from build123d import *

# Parameters (mm, degrees)
F0_R     = 50
F1_DEPTH = 6
F2_R     = 3
F3_DEPTH = 6.001
F4_R     = 4
F5_DEPTH = 6.001


with BuildPart() as f1:
    # F0 (on Front) → F1 (new body)
    with BuildSketch(Plane.XZ):
        Circle(F0_R)
    extrude(amount=F1_DEPTH)

    # F2 (on face) → F3 (cut, through all)
    with BuildSketch(Plane.XZ.offset(6)):
        Circle(F2_R)
    extrude(amount=-F3_DEPTH, mode=Mode.SUBTRACT)

    # F4 (on face) → F5 (cut, through all)
    with BuildSketch(Plane.XZ.offset(6)):
        with Locations((0, 38)):
            Circle(F4_R)
        with Locations((-22.33584, -30.742646)):
            Circle(F4_R)
        with Locations((-36.140148, 11.742646)):
            Circle(F4_R)
        with Locations((22.33584, -30.742646)):
            Circle(F4_R)
        with Locations((36.140148, 11.742646)):
            Circle(F4_R)
    extrude(amount=-F5_DEPTH, mode=Mode.SUBTRACT)


solid = f1.part
Verification items for the finished model (mm, model axes). Coordinates: 2 decimals unless noted, no trailing zeros. Order: outer loops, then holes, each group sorted by start corner. A loop starts at its lowest first (then second) coordinate and runs counter-clockwise, first axis right, second up. Notation, with made-up numbers: (-35.5, 3.25) -> (-17.5, 3.25) arc R20 cw to (-17.5, 17.25) -> close; hole circle Ø10 at (-15, 44). An arc over 180 degrees is marked (long way). Use CSV: the item, a comma, the result in double quotes. Start each with the question number.
Q1. Section check D-D, the plane y = -2.4. Record the cut outline in (x, z), and give its area (3 significant figures).
Q2. Section check B-B, the plane z = 0. Record the cut outline in (x, y), and give its area (3 significant figures).
Q3. Section check C-C, the plane x = -24.5. Record the cut outline in (y, z).
Q4. Depth check by flat-ended pin: P1, Ø2, axis at x = -10.5, y = -1, coming from the -Z side; P2, Ø2, axis at x = 32.5, y = -3.5, coming from the +Z side; P3, Ø2, axis at y = -1.5, z = -14, coming from the -X side. Enter the tip coordinate at first touch or a pass-through.
Q5. Thickness scan on line 1 along X through (y, z) = (-4.4, 13); line 2 along Z through (x, y) = (-37.5, -4.45); line 3 along X through (y, z) = (-1.05, 37). Record the ranges inside material, lowest first.
Q6. Draft check along X on faces 1 (the cylindrical face through (21.469, -3.042, -34.648)), 2 (the flat face through (10, -6, 1)), 3 (the cylindrical face through (47.69, -2.96, 15.02)). Enter one of: +X half, -X half, draft (parallel to the pull), parting line (faces both ways), or undercut.
Q7. Section check A-A, the plane x = 0. Record the cut outline in (y, z).
Returned:
1,outline,"circle Ø100 at (0, 0); hole circle Ø8 at (-36.14, 11.74); hole circle Ø8 at (-22.34, -30.74); hole circle Ø8 at (0, 38); hole circle Ø6 at (0, 0); hole circle Ø8 at (22.34, -30.74); hole circle Ø8 at (36.14, 11.74)"
1,area,"7,570 mm^2"
2,outline,"(-50, -6) -> (-3, -6) -> (-3, 0) -> (-50, 0) -> close; (3, -6) -> (50, -6) -> (50, 0) -> (3, 0) -> close"
2,area,"564 mm^2"
3,outline,"(-6, -43.59) -> (0, -43.59) -> (0, -34.11) -> (-6, -34.11) -> close; (-6, -27.38) -> (0, -27.38) -> (0, 43.59) -> (-6, 43.59) -> close"
4,P1,"stops at z = -49.09"
4,P2,"stops at z = 38.83"
4,P3,"stops at x = -48.28"
5,line 1,"x = -48.28 to -39.94, -32.34 to 32.34, 39.94 to 48.28"
5,line 2,"z = -33.07 to 7.98, 15.5 to 33.07"
5,line 3,"x = -33.63 to -3.87, 3.87 to 33.63"
6,face 1,"undercut"
6,face 2,"draft"
6,face 3,"parting line"
7,outline,"(-6, -50) -> (0, -50) -> (0, -3) -> (-6, -3) -> close; (-6, 3) -> (0, 3) -> (0, 34) -> (-6, 34) -> close; (-6, 42) -> (0, 42) -> (0, 50) -> (-6, 50) -> close"
